For this review, take the finished solid that the model builds, in its own axes (mm). A direction names the side the tool comes from. Give positions to 0.01 mm unless a question says otherwise; leave off trailing zeros. Loops run counter-clockwise (first coordinate to the right, second up) from the corner with the lowest first, then second, coordinate; pieces in that order, holes last. Notation, with made-up numbers: (0, 24) -> (36, 24) arc R17 ccw to (36, 36) -> close; hole circle Ø9 at (63.5, 33.25). An arc over 180 degrees is marked (long way). Answer as CSV lines item,"result". Start each with the question number.
Item 1: For L1, parallel to Z at x = 9.75, y = 44.47; L2, parallel to Y at x = 22, z = -33.5; L3, parallel to Y at x = 10.75, z = -18.5, list the stretches that pass through material, from the lowest coordinate up. Write a range as from..to.
Item 2: Add section C-C on x = 24.5. State the section outline as (y, z) points.
Item 3: The part is to be moulded in two halves that separate along X. For faces 1 (the face through (23, 25, -32)), 2 (the face through (16.54, 15.96, -38.47)), 3 (the face through (9, -2.5, -49)), say which applies: +X half, -X half, draft (parallel to the pull), parting line (faces both ways), or undercut.
Item 4: Add section D-D on z = -16. State the section outline as (x, y) points.
Item 5: Add section A-A on x = 11.5. State the section outline as (y, z) points.
Item 6: Machinability: for faces 4 (the face through (11, 32, -41.312)), 5 (the face through (1, 18.5, -39)), 6 (the face through (11.339, 20.138, -69.778)), 7 (the face through (24.77, 19.4, -26.23)), which of the approach directions +Z, -Z, +X, -X, +Y, -Y give a long, thin tool a straight path to every point of the face, cutting with its end or side? Answer none if there is none.
Item 7: Clearance check with flat-ended pins moving along their axes: P1, Ø3, axis at x = 14.5, y = 28, coming from the +Z side; P2, Ø6.5, axis at x = 16, z = -35, coming from the -Y side; P3, Ø12, axis at y = 21, z = -33.5, coming from the -X side; P4, Ø2, axis at x = 23, y = 17, coming from the -Z side. State where each tip first meets the part, or that it passes through.
Item 8: Add section B-B on y = 44.47. State the section outline as (x, z) points, plus the area to 4 significant figures.
Autodesk Inventor part; units mm, degrees
ref_plane "Arbeitsebene1" through (26.5, 0, 0) normal (1, 0, 0) x (0, 0, -1)
ref_plane "YZ Plane" through (0, 0, 0) normal (1, 0, 0) x (0, 1, 0)
ref_plane "XZ Plane" through (0, 0, 0) normal (0, 1, 0) x (-1, 0, 0)
sketch "Skizze1" plane through (0, 0, 0) normal (1, 0, 0) x (0, 1, 0)
  line L0 (0, 0) -> (0, -100)
  line L1 (0, -100) -> (41.1159, -51)
  line L2 (0, 0) -> (41.1159, -49)
  circle A0 centre (44.47, -50) radius 3.5
  circle A1 centre (44.47, -50) radius 1.75
  dimension "d0" = 40
  dimension "d1" = 3.5
  dimension "d2" = 7
  dimension "d3" = 2
  dimension "d4" = 100
extrude "Extrusion1" add sketch "Skizze1" along normal blind 28.5
sketch "Skizze2" plane through (0, 0, -100) normal (0, -1, 0) x (1, 0, 0)
  line L0 (0, 100) -> (0, 0)
  line L1 (0, 0) -> (28.5, 0)
  line L2 (28.5, 100) -> (28.5, 0)
  line L3 (0, 100) -> (28.5, 100)
extrude "Extrusion2" add sketch "Skizze2" along normal blind 5
sketch "Skizze3" plane through (28.5, 0, 0) normal (1, 0, 0) x (0, 0, -1)
  line L0 (100, 0) -> (51, 41.1159)
  arc A0 (51, 41.1159) -> (49, 41.1159) centre (50, 44.47) ccw
  line L1 (49, 41.1159) -> (0, 0)
  line L2 (0, 0) -> (0, -5)
  line L3 (100, -5) -> (0, -5)
  line L4 (100, 0) -> (100, -5)
  circle A1 centre (50, 44.47) radius 1.75
  line L5 (49, 41.1159) -> (0, 0)
  line L6 (0, 0) -> (100, 0)
  line L7 (0, 0) -> (0, -5)
  line L8 (0, -2.5) -> (100, -2.5)
extrude "Extrusion3" cut sketch "Skizze3" against normal blind 24 contours L4 L8 L2 L6
sketch "Skizze4" plane through (28.5, 0, 0) normal (1, 0, 0) x (0, 0, -1)
  line L0 (0, 0) -> (100, 0)
  line L1 (100, -5) -> (0, -5)
  line L2 (0, 0) -> (13.75, 0)
  line L3 (13.75, 0) -> (13.75, -5)
  line L4 (13.75, -5) -> (0, -5)
  line L5 (0, -5) -> (0, 0)
  line L6 (100, 0) -> (51, 41.1159)
  line L7 (100, 0) -> (86.25, 0)
  line L8 (86.25, 0) -> (86.25, -5)
  line L9 (86.25, -5) -> (100, -5)
  line L10 (100, -5) -> (100, 0)
  dimension "d11" = 72.5
extrude "Extrusion4" cut sketch "Skizze4" against normal through all contours L0 L3 L1 L5 | L0 L10 L1 L8
sketch "Skizze5" plane through (28.5, 0, 0) normal (1, 0, 0) x (0, 0, -1)
  line L0 (86.25, -5) -> (86.25, -2.5)
  line L1 (86.25, -2.5) -> (13.75, -2.5)
  line L2 (13.75, -2.5) -> (13.75, -5)
  line L3 (86.25, -5) -> (13.75, -5)
  point P0 (0, 0)
extrude "Extrusion5" cut sketch "Skizze5" against normal blind 14.5
ref_plane "Arbeitsebene1" through (26.5, 0, 0) normal (1, 0, 0) x (0, 0, -1)
sketch "Skizze6" plane through (26.5, 0, 0) normal (1, 0, 0) x (0, 0, -1)
  line L0 (49, 41.1159) -> (0, 0)
  line L1 (100, 0) -> (51, 41.1159)
  line L2 (13.75, 0) -> (0, 0)
  line L3 (13.75, 0) -> (86.25, 0)
  line L4 (100, 0) -> (86.25, 0)
  line L5 (3.1114, 0) -> (50, 39.3442)
  line L6 (50, 39.3442) -> (96.8886, 0)
  circle A0 centre (50, 44.47) radius 1.75
  dimension "d17" = 2
extrude "Extrusion6" cut sketch "Skizze6" against normal blind 3.5 contours L2 L5 L6 L4 L3
sketch "Skizze7" plane through (23, 0, 0) normal (1, 0, 0) x (0, 0, -1)
  line L0 (96.8886, 0) -> (3.1114, 0)
  line L1 (50, 39.3442) -> (96.8886, 0)
  line L2 (3.1114, 0) -> (50, 39.3442)
  line L3 (96.8886, 0) -> (3.1114, 0)
  line L4 (6.2229, 0) -> (50, 36.7334)
  line L5 (50, 36.7334) -> (93.7771, 0)
  line L6 (100, 0) -> (86.25, 0)
  point P0 (0, 0)
  dimension "d20" = 2
extrude "Extrusion7" cut sketch "Skizze7" along normal through all contours L0 L4 L5
sketch "Skizze8" plane through (0, 0, 0) normal (-1, 0, 0) x (0, 0, 1)
  line L0 (-100, 0) -> (-86.25, 0)
  line L1 (-13.75, 0) -> (0, 0)
  line L2 (-13.75, 0) -> (-86.25, 0)
  line L3 (-49, 41.1159) -> (0, 0)
  line L4 (-100, 0) -> (-51, 41.1159)
  circle A0 centre (-50, 44.47) radius 1.75
  line L5 (-93.7771, 0) -> (-96.8886, 0)
  line L6 (-50, 39.3442) -> (-96.8886, 0)
  line L7 (-92.1215, 4) -> (-7.8785, 4)
  line L8 (-3.1114, 0) -> (-50, 39.3442)
  line L9 (-93.7771, 0) -> (-50, 36.7334)
  line L10 (-50, 36.7334) -> (-6.2229, 0)
  point P0 (-10.9899, 4)
  point P1 (-89.0101, 4)
  dimension "d23" = 4
extrude "Extrusion8" cut sketch "Skizze8" against normal up to surface (23 mm away) contours L9 L10 L7
sketch "Skizze9" plane through (0, 0, 0) normal (-1, 0, 0) x (0, 0, 1)
  line L0 (-89.0101, 4) -> (-50, 36.7334)
  line L1 (-50, 36.7334) -> (-10.9899, 4)
  line L2 (-10.9899, 4) -> (-89.0101, 4)
  line L3 (-86.25, 0) -> (-86.25, -5)
  line L4 (-13.75, -5) -> (-86.25, -5)
  line L5 (-13.75, -5) -> (-13.75, 0)
  line L6 (-13.75, 0) -> (0, 0)
  line L7 (-49, 41.1159) -> (0, 0)
  arc A0 (-49, 41.1159) -> (-51, 41.1159) centre (-50, 44.47) ccw
  line L8 (-100, 0) -> (-51, 41.1159)
  line L9 (-100, 0) -> (-86.25, 0)
  circle A1 centre (-50, 44.47) radius 1.75
  line L10 (-19.9281, 11.5) -> (-41.3116, 11.5)
  line L11 (-41.3116, 11.5) -> (-41.3116, 13.5)
  line L12 (-41.3116, 13.5) -> (-22.3116, 13.5)
  line L13 (-50, 36.7334) -> (-10.9899, 4)
  point P0 (-30.495, 20.3667)
  dimension "d26" = 2
  dimension "d27" = 19
  dimension "d38" = 7.5
extrude "Extrusion9" add sketch "Skizze9" against normal up to surface (23 mm away) contours L1 L10 L11 L12
sketch "Skizze10" plane through (0, 13.5, -22.3116) normal (0, 1, 0) x (1, 0, 0)
  line L0 (23, 19) -> (23, 0)
  line L1 (0, 19) -> (23, 19)
  line L2 (0, 0) -> (0, 19)
  line L3 (23, 0) -> (0, 0)
  circle A0 centre (16, 17) radius 1
  circle A1 centre (1, 17) radius 1
  point P0 (0, -22.3116)
  dimension "d30" = 2
  dimension "d31" = 15
  dimension "d32" = 2
  dimension "d39" = 1
extrude "Extrusion10" cut sketch "Skizze10" along normal through all contours A1 | L0 L3 L2 L1 | A0
extrude "Extrusion11" add sketch "Skizze10" along normal blind 5 contours A1 | A0
equation "\"d32\" = d30"
properties part number "roof_foot"
Computed values:
1,L1,"-53.5..-51.75, -48.25..-46.5"
1,L2,"0..4, 11.5..13.5"
1,L3,"-5..-2.5, 0..4, 10.3..15.52"
2,outline,"(0, -100) -> (41.12, -51) arc R3.5 ccw (long way) to (41.12, -49) -> (0, 0) -> (0, -3.11) -> (39.34, -50) -> (0, -96.89) -> close; hole circle Ø3.5 at (44.47, -50)"
3,face 1,"-X half"
3,face 2,"undercut"
3,face 3,"draft"
4,outline,"(0, -5) -> (14, -5) -> (14, -2.5) -> (4.5, -2.5) -> (4.5, 0) -> (23, 0) -> (23, 4) -> (0, 4) -> close; (0, 8.2) -> (23, 8.2) -> (23, 10.81) -> (26.5, 10.81) -> (26.5, 8.2) -> (28.5, 8.2) -> (28.5, 13.43) -> (0, 13.43) -> close"
5,outline,"(-5, -86.25) -> (-2.5, -86.25) -> (-2.5, -13.75) -> (-5, -13.75) -> close; (0, -100) -> (41.12, -51) arc R3.5 ccw (long way) to (41.12, -49) -> (34.66, -41.31) -> (29.44, -41.31) -> (36.73, -50) -> (4, -89.01) -> (4, -10.99) -> (11.5, -19.93) -> (11.5, -41.31) -> (13.5, -41.31) -> (13.5, -22.31) -> (18.72, -22.31) -> (0, 0) -> close; hole circle Ø3.5 at (44.47, -50)"
6,face 4,"+Z, -X, +Y"
6,face 5,"+X, -X, +Y"
6,face 6,"+X, -X"
6,face 7,"-Y"
7,P1,"z = -41.31"
7,P2,"y = -5"
7,P3,"x = 0.07"
7,P4,"z = -80.93"
8,outline,"(0, -53.5) -> (28.5, -53.5) -> (28.5, -51.75) -> (0, -51.75) -> close; (0, -48.25) -> (28.5, -48.25) -> (28.5, -46.5) -> (0, -46.5) -> close"
8,area,"99.75 mm²"
